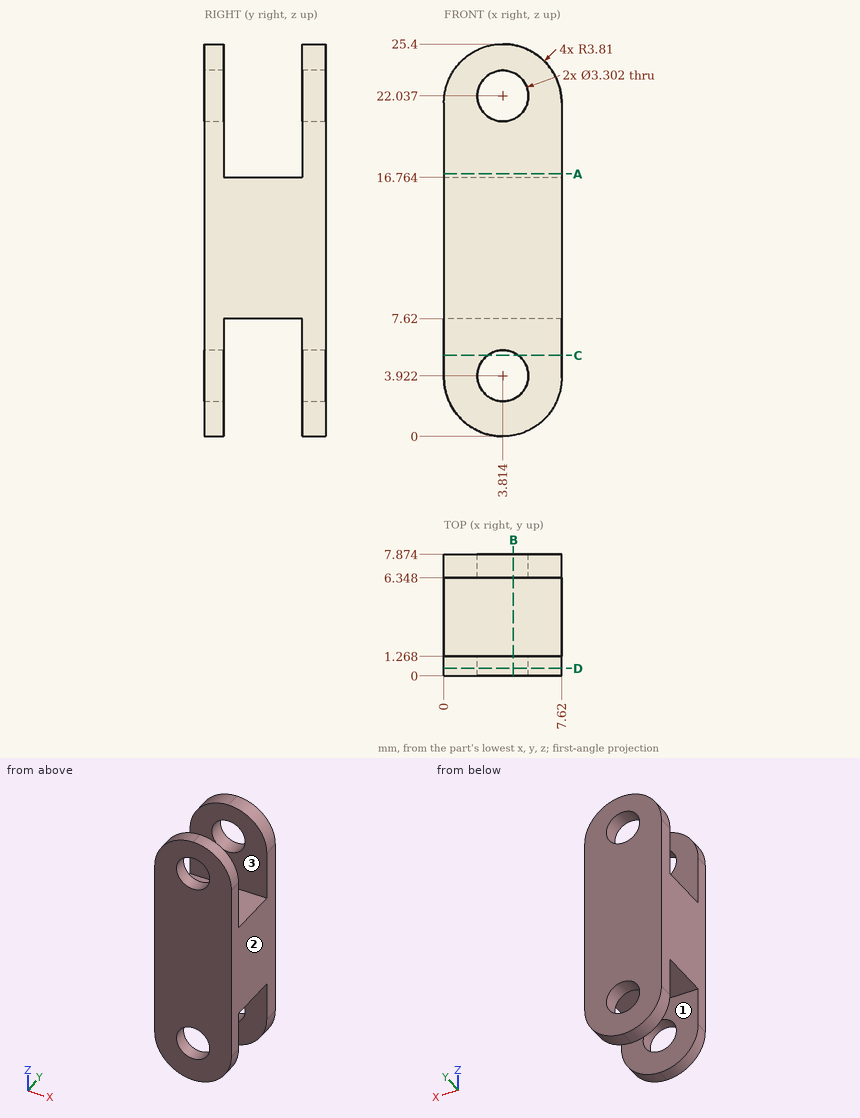
Design review of the part shown in the three views and the two pictorial views. Dimensions are in mm from the part's minimum x, y and z. A direction names the side the tool comes from. Round coordinates to 2 decimals unless told otherwise and drop trailing zeros. Loops run counter-clockwise (first coordinate to the right, second up) from the corner with the lowest first, then second, coordinate; pieces in that order, holes last. Notation, with made-up numbers: (10.25, -11.5) - (24.25, -11.5) arc R21 cw to (24.25, 20.5) - close; hole circle Ø6 at (-33, 80.25). An arc over 180 degrees is marked (long way). Answer as CSV lines item,"result".
(1) Consider section B-B on x = 4.5. Give the boundary of the cut face in (y, z) (1 decimal).
Checked values:
outline,"(0, 0.1) - (1.3, 0.1) - (1.3, 2.4) - (0, 2.4) - close; (0, 5.4) - (1.3, 5.4) - (1.3, 7.6) - (6.3, 7.6) - (6.3, 5.4) - (7.9, 5.4) - (7.9, 20.5) - (6.3, 20.5) - (6.3, 16.8) - (1.3, 16.8) - (1.3, 20.5) - (0, 20.5) - close; (0, 23.5) - (1.3, 23.5) - (1.3, 25.3) - (0, 25.3) - close; (6.3, 0.1) - (7.9, 0.1) - (7.9, 2.4) - (6.3, 2.4) - close; (6.3, 23.5) - (7.9, 23.5) - (7.9, 25.3) - (6.3, 25.3) - close"
(2) Consider section D-D on y = 0.5. Give the number of separate pieces and of enclosed holes in the cut face, then the cut area to 3 significant figures.
Checked values:
separate pieces,"1"
enclosed holes,"2"
area,"164 mm2"
(3) Insertion check: P1, Ø1.5, axis at x = 2.5, y = 4.5, coming from the +Z side; P2, Ø2, axis at x = 3.81, z = 3.92, coming from the +Y side; P3, Ø2, axis at x = 4, y = 4.5, coming from the -Z side. Each pin has a flat end and moves straight along its axis. Give the tip position at first contact, or say it passes through.
Checked values:
P1,"stops at z = 16.76"
P2,"passes through"
P3,"stops at z = 7.62"
(4) Wall thickness on line 1 (Y direction, x = 6.5, z = 7); line 2 (Z direction, x = 2.5, y = 0.5) (1 decimal); line 3 (X direction, y = 6.75, z = 22.25): over which ranges is each line inside the solid? List them lowest first.
Checked values:
line 1,"y = 0 to 1.27, 6.35 to 7.87"
line 2,"z = 0.2 to 2.9, 4.9 to 21, 23 to 25.2"
line 3,"x = 0.06 to 2.18, 5.45 to 7.56"
(5) Consider section C-C on z = 5.25. Give the boundary of the cut face in (x, y) (1 decimal), then the cut area to 3 significant figures.
Checked values:
outline,"(0, 0) - (2.8, 0) - (2.8, 1.3) - (0, 1.3) - close; (0, 6.3) - (2.8, 6.3) - (2.8, 7.9) - (0, 7.9) - close; (4.8, 0) - (7.6, 0) - (7.6, 1.3) - (4.8, 1.3) - close; (4.8, 6.3) - (7.6, 6.3) - (7.6, 7.9) - (4.8, 7.9) - close"
area,"15.8 mm2"
(6) Consider section A-A on z = 17. Give the boundary of the cut face in (x, y).
Checked values:
outline,"(0, 0) - (7.62, 0) - (7.62, 1.27) - (0, 1.27) - close; (0, 6.35) - (7.62, 6.35) - (7.62, 7.87) - (0, 7.87) - close"
(7) Tool access review of the marked faces 1, 2 and 3: name each direction out of +Z, -Z, +X, -X, +Y, -Y from which nothing blocks a thin tool from reaching the whole face with its end or side.
Checked values:
face 1,"-Z, +X, -X"
face 2,"+Z, -Z, +X, +Y, -Y"
face 3,"+Z, +X, -X"
